```python
from build123d import *

# Parameters (mm, degrees)
SKETCH_1_W             = 891
SKETCH_1_H             = 1135
SKETCH_1_R             = 2.25
SM_BASE_FLANGE_1_DEPTH = 2
CUT_EXTRUDE_1_REACH    = 1444.952
SKETCH_7_W             = 294.359434409
SKETCH_7_H             = 100
CUT_EXTRUDE_2_REACH    = 1444.952
SKETCH_8_R             = 5
CUT_EXTRUDE_3_REACH    = 1444.952
SKETCH_9_W             = 45
SKETCH_9_H             = 45
CUT_EXTRUDE_4_REACH    = 1444.952
SKETCH_10_R            = 2.5


# Sheet-metal steps are written as plain solids
with BuildPart() as part:
    # Sketch 1 → Базовая кромка1 (new body)
    with BuildSketch(Plane.XY):
        with Locations((445.5, 567.5)):
            Rectangle(SKETCH_1_W, SKETCH_1_H)
        with Locations((285.5, 912)):
            Circle(SKETCH_1_R, mode=Mode.SUBTRACT)
        with Locations((285.5, 704)):
            Circle(SKETCH_1_R, mode=Mode.SUBTRACT)
        with Locations((285.5, 496)):
            Circle(SKETCH_1_R, mode=Mode.SUBTRACT)
        with Locations((285.5, 288)):
            Circle(SKETCH_1_R, mode=Mode.SUBTRACT)
        with Locations((285.5, 80)):
            Circle(SKETCH_1_R, mode=Mode.SUBTRACT)
        with Locations((445.5, 80)):
            Circle(SKETCH_1_R, mode=Mode.SUBTRACT)
        with Locations((605.5, 80)):
            Circle(SKETCH_1_R, mode=Mode.SUBTRACT)
        with Locations((605.5, 288)):
            Circle(SKETCH_1_R, mode=Mode.SUBTRACT)
        with Locations((605.5, 496)):
            Circle(SKETCH_1_R, mode=Mode.SUBTRACT)
        with Locations((605.5, 704)):
            Circle(SKETCH_1_R, mode=Mode.SUBTRACT)
        with Locations((605.5, 912)):
            Circle(SKETCH_1_R, mode=Mode.SUBTRACT)
        with Locations((605.5, 1120)):
            Circle(SKETCH_1_R, mode=Mode.SUBTRACT)
        with Locations((445.5, 1120)):
            Circle(SKETCH_1_R, mode=Mode.SUBTRACT)
        with Locations((285.5, 1120)):
            Circle(SKETCH_1_R, mode=Mode.SUBTRACT)
    extrude(amount=-SM_BASE_FLANGE_1_DEPTH)

    # Эскиз7 → Вырез-Вытянуть1 (cut, up to next)
    with BuildSketch(Plane(origin=(0, 0, -2), x_dir=(-1, 0, 0), z_dir=(0, 0, -1)), mode=Mode.PRIVATE) as cut_extrude_1_sk1:
        with Locations((-445.494464103, 990)):
            Rectangle(SKETCH_7_W, SKETCH_7_H)
    cut_extrude_1_tool1 = extrude(cut_extrude_1_sk1.sketch, amount=-CUT_EXTRUDE_1_REACH, mode=Mode.PRIVATE) & part.part
    add(cut_extrude_1_tool1.solids().sort_by_distance((445.494464, 990, -2))[0], mode=Mode.SUBTRACT)

    # Эскиз8 → Вырез-Вытянуть2 (cut, up to next)
    with BuildSketch(Plane(origin=(0, 0, -2), x_dir=(-1, 0, 0), z_dir=(0, 0, -1)), mode=Mode.PRIVATE) as cut_extrude_2_sk1:
        with Locations((-36.893974432, 567.5)):
            Circle(SKETCH_8_R)
    cut_extrude_2_tool1 = extrude(cut_extrude_2_sk1.sketch, amount=-CUT_EXTRUDE_2_REACH, mode=Mode.PRIVATE) & part.part
    # Эскиз8 → Вырез-Вытянуть2 (cut, up to next)
    with BuildSketch(Plane(origin=(0, 0, -2), x_dir=(-1, 0, 0), z_dir=(0, 0, -1)), mode=Mode.PRIVATE) as cut_extrude_2_sk2:
        with Locations((-854.014883074, 567.5)):
            Circle(SKETCH_8_R)
    cut_extrude_2_tool2 = extrude(cut_extrude_2_sk2.sketch, amount=-CUT_EXTRUDE_2_REACH, mode=Mode.PRIVATE) & part.part
    add(cut_extrude_2_tool1.solids().sort_by_distance((36.893974, 567.5, -2))[0], mode=Mode.SUBTRACT)
    add(cut_extrude_2_tool2.solids().sort_by_distance((854.014883, 567.5, -2))[0], mode=Mode.SUBTRACT)

    # Эскиз9 → Вырез-Вытянуть3 (cut, up to next)
    with BuildSketch(Plane.XY, mode=Mode.PRIVATE) as cut_extrude_3_sk1:
        with Locations((609.814746898, 602.5)):
            Rectangle(SKETCH_9_W, SKETCH_9_H)
    cut_extrude_3_tool1 = extrude(cut_extrude_3_sk1.sketch, amount=-CUT_EXTRUDE_3_REACH, mode=Mode.PRIVATE) & part.part
    add(cut_extrude_3_tool1.solids().sort_by_distance((609.814747, 602.5, 0))[0], mode=Mode.SUBTRACT)

    # Эскиз10 → Вырез-Вытянуть4 (cut, up to next)
    with BuildSketch(Plane(origin=(0, 0, -2), x_dir=(-1, 0, 0), z_dir=(0, 0, -1)), mode=Mode.PRIVATE) as cut_extrude_4_sk1:
        with Locations((-854.094953773, 1120)):
            Circle(SKETCH_10_R)
    cut_extrude_4_tool1 = extrude(cut_extrude_4_sk1.sketch, amount=-CUT_EXTRUDE_4_REACH, mode=Mode.PRIVATE) & part.part
    # Эскиз10 → Вырез-Вытянуть4 (cut, up to next)
    with BuildSketch(Plane(origin=(0, 0, -2), x_dir=(-1, 0, 0), z_dir=(0, 0, -1)), mode=Mode.PRIVATE) as cut_extrude_4_sk2:
        with Locations((-854.094953773, 912)):
            Circle(SKETCH_10_R)
    cut_extrude_4_tool2 = extrude(cut_extrude_4_sk2.sketch, amount=-CUT_EXTRUDE_4_REACH, mode=Mode.PRIVATE) & part.part
    # Эскиз10 → Вырез-Вытянуть4 (cut, up to next)
    with BuildSketch(Plane(origin=(0, 0, -2), x_dir=(-1, 0, 0), z_dir=(0, 0, -1)), mode=Mode.PRIVATE) as cut_extrude_4_sk3:
        with Locations((-854.094953773, 704)):
            Circle(SKETCH_10_R)
    cut_extrude_4_tool3 = extrude(cut_extrude_4_sk3.sketch, amount=-CUT_EXTRUDE_4_REACH, mode=Mode.PRIVATE) & part.part
    # Эскиз10 → Вырез-Вытянуть4 (cut, up to next)
    with BuildSketch(Plane(origin=(0, 0, -2), x_dir=(-1, 0, 0), z_dir=(0, 0, -1)), mode=Mode.PRIVATE) as cut_extrude_4_sk4:
        with Locations((-854.094953773, 496)):
            Circle(SKETCH_10_R)
    cut_extrude_4_tool4 = extrude(cut_extrude_4_sk4.sketch, amount=-CUT_EXTRUDE_4_REACH, mode=Mode.PRIVATE) & part.part
    # Эскиз10 → Вырез-Вытянуть4 (cut, up to next)
    with BuildSketch(Plane(origin=(0, 0, -2), x_dir=(-1, 0, 0), z_dir=(0, 0, -1)), mode=Mode.PRIVATE) as cut_extrude_4_sk5:
        with Locations((-854.094953773, 288)):
            Circle(SKETCH_10_R)
    cut_extrude_4_tool5 = extrude(cut_extrude_4_sk5.sketch, amount=-CUT_EXTRUDE_4_REACH, mode=Mode.PRIVATE) & part.part
    # Эскиз10 → Вырез-Вытянуть4 (cut, up to next)
    with BuildSketch(Plane(origin=(0, 0, -2), x_dir=(-1, 0, 0), z_dir=(0, 0, -1)), mode=Mode.PRIVATE) as cut_extrude_4_sk6:
        with Locations((-854.094953773, 80)):
            Circle(SKETCH_10_R)
    cut_extrude_4_tool6 = extrude(cut_extrude_4_sk6.sketch, amount=-CUT_EXTRUDE_4_REACH, mode=Mode.PRIVATE) & part.part
    # Эскиз10 → Вырез-Вытянуть4 (cut, up to next)
    with BuildSketch(Plane(origin=(0, 0, -2), x_dir=(-1, 0, 0), z_dir=(0, 0, -1)), mode=Mode.PRIVATE) as cut_extrude_4_sk7:
        with Locations((-36.893974432, 1120)):
            Circle(SKETCH_10_R)
    cut_extrude_4_tool7 = extrude(cut_extrude_4_sk7.sketch, amount=-CUT_EXTRUDE_4_REACH, mode=Mode.PRIVATE) & part.part
    # Эскиз10 → Вырез-Вытянуть4 (cut, up to next)
    with BuildSketch(Plane(origin=(0, 0, -2), x_dir=(-1, 0, 0), z_dir=(0, 0, -1)), mode=Mode.PRIVATE) as cut_extrude_4_sk8:
        with Locations((-36.893974432, 912)):
            Circle(SKETCH_10_R)
    cut_extrude_4_tool8 = extrude(cut_extrude_4_sk8.sketch, amount=-CUT_EXTRUDE_4_REACH, mode=Mode.PRIVATE) & part.part
    # Эскиз10 → Вырез-Вытянуть4 (cut, up to next)
    with BuildSketch(Plane(origin=(0, 0, -2), x_dir=(-1, 0, 0), z_dir=(0, 0, -1)), mode=Mode.PRIVATE) as cut_extrude_4_sk9:
        with Locations((-36.893974432, 704)):
            Circle(SKETCH_10_R)
    cut_extrude_4_tool9 = extrude(cut_extrude_4_sk9.sketch, amount=-CUT_EXTRUDE_4_REACH, mode=Mode.PRIVATE) & part.part
    # Эскиз10 → Вырез-Вытянуть4 (cut, up to next)
    with BuildSketch(Plane(origin=(0, 0, -2), x_dir=(-1, 0, 0), z_dir=(0, 0, -1)), mode=Mode.PRIVATE) as cut_extrude_4_sk10:
        with Locations((-36.893974432, 496)):
            Circle(SKETCH_10_R)
    cut_extrude_4_tool10 = extrude(cut_extrude_4_sk10.sketch, amount=-CUT_EXTRUDE_4_REACH, mode=Mode.PRIVATE) & part.part
    # Эскиз10 → Вырез-Вытянуть4 (cut, up to next)
    with BuildSketch(Plane(origin=(0, 0, -2), x_dir=(-1, 0, 0), z_dir=(0, 0, -1)), mode=Mode.PRIVATE) as cut_extrude_4_sk11:
        with Locations((-36.893974432, 288)):
            Circle(SKETCH_10_R)
    cut_extrude_4_tool11 = extrude(cut_extrude_4_sk11.sketch, amount=-CUT_EXTRUDE_4_REACH, mode=Mode.PRIVATE) & part.part
    # Эскиз10 → Вырез-Вытянуть4 (cut, up to next)
    with BuildSketch(Plane(origin=(0, 0, -2), x_dir=(-1, 0, 0), z_dir=(0, 0, -1)), mode=Mode.PRIVATE) as cut_extrude_4_sk12:
        with Locations((-36.893974432, 80)):
            Circle(SKETCH_10_R)
    cut_extrude_4_tool12 = extrude(cut_extrude_4_sk12.sketch, amount=-CUT_EXTRUDE_4_REACH, mode=Mode.PRIVATE) & part.part
    add(cut_extrude_4_tool1.solids().sort_by_distance((854.094954, 1120, -2))[0], mode=Mode.SUBTRACT)
    add(cut_extrude_4_tool2.solids().sort_by_distance((854.094954, 912, -2))[0], mode=Mode.SUBTRACT)
    add(cut_extrude_4_tool3.solids().sort_by_distance((854.094954, 704, -2))[0], mode=Mode.SUBTRACT)
    add(cut_extrude_4_tool4.solids().sort_by_distance((854.094954, 496, -2))[0], mode=Mode.SUBTRACT)
    add(cut_extrude_4_tool5.solids().sort_by_distance((854.094954, 288, -2))[0], mode=Mode.SUBTRACT)
    add(cut_extrude_4_tool6.solids().sort_by_distance((854.094954, 80, -2))[0], mode=Mode.SUBTRACT)
    add(cut_extrude_4_tool7.solids().sort_by_distance((36.893974, 1120, -2))[0], mode=Mode.SUBTRACT)
    add(cut_extrude_4_tool8.solids().sort_by_distance((36.893974, 912, -2))[0], mode=Mode.SUBTRACT)
    add(cut_extrude_4_tool9.solids().sort_by_distance((36.893974, 704, -2))[0], mode=Mode.SUBTRACT)
    add(cut_extrude_4_tool10.solids().sort_by_distance((36.893974, 496, -2))[0], mode=Mode.SUBTRACT)
    add(cut_extrude_4_tool11.solids().sort_by_distance((36.893974, 288, -2))[0], mode=Mode.SUBTRACT)
    add(cut_extrude_4_tool12.solids().sort_by_distance((36.893974, 80, -2))[0], mode=Mode.SUBTRACT)


solid = part.part
```
CAD build for the part. Positions are in the model's coordinates, mm. Coordinates: 2 decimals unless noted, no trailing zeros. Order: outer loops, then holes, each group sorted by start corner. A loop starts at its lowest first (then second) coordinate and runs counter-clockwise, first axis right, second up. Notation, with made-up numbers: M 51,-4 L 65,-4 A24 ccw 65,19 Z; hole C -34,51 d10. An arc over 180 degrees is marked long. Write each question's results on one line, items separated by ' | '. Start each with the question number.
Q1. Flat gauge pin, fed straight in: P1, Ø3.5, axis at x = 285.5, y = 704, coming from the -Z side. Where does the tip first touch, or does it go through?
Q2. Cut at A-A (x = 324). List the corners of the cut face in (y, z).
Q3. Cut at B-B (z = -0.5). Count the separate pieces of the cut face and the enclosed holes in it, then the cut area to 3 significant figures.
Q4. Drill centre lines: probe 1 along X at (y, z) = (496, -0.5); probe 2 along X at (y, z) = (964.5, -0.05). Where is each one in solid material? Low to high. Write a range as from..to.
Found:
1) P1: through
2) outline: M 0,-2 L 940,-2 L 940,0 L 0,0 Z; M 1040,-2 L 1135,-2 L 1135,0 L 1040,0 Z
3) separate pieces: 1 | enclosed holes: 30 | area: 979,000 mm²
4) probe 1: 0..34.39, 39.39..283.25, 287.75..603.25, 607.75..851.59, 856.59..891 | probe 2: 0..298.31, 592.67..891
